Here's how the part is built. I have some questions about the finished solid (model axes, mm). Face numbers are marked on the shaded views. A direction names the side the tool comes from. Round coordinates to 2 decimals unless told otherwise and drop trailing zeros. Write each loop counter-clockwise with the first axis right and the second up, starting at its lowest first coordinate (ties: lowest second). Pieces come first, ordered by that corner, then holes. Notation, with made-up numbers: (-29, -24.75) - (1, -24.75) arc R27 cw to (1, 2.25) - close; hole circle Ø3 at (9.25, 58). An arc over 180 degrees is marked (long way). Return JSON: item names as keys, results as strings. Group by question number.
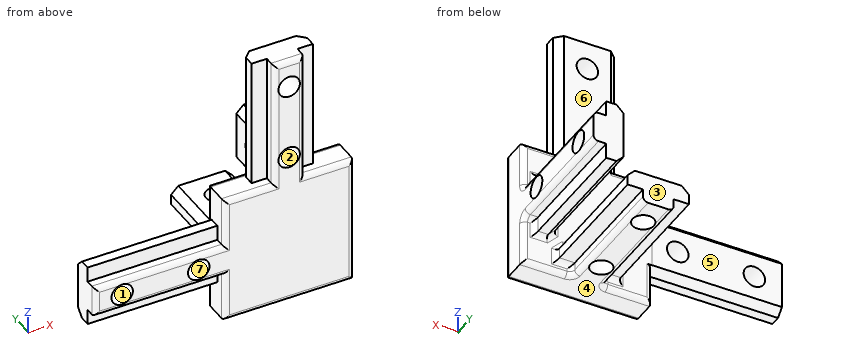
```python
from build123d import *

# Parameters (mm, degrees)
SKETCH1_W             = 25.4
SKETCH1_H             = 25.4
BOSS_EXTRUDE1_DEPTH   = 5.91
BOSS_EXTRUDE2_DEPTH   = 25.4
BOSS_EXTRUDE3_DEPTH   = 25.4
BOSS_EXTRUDE4_DEPTH   = 25.4
FILLET2_R             = 1
M5X0_8_TAPPED_HOLE2_D = 4.2
M5X0_8_TAPPED_HOLE3_D = 4.2
M5X0_8_TAPPED_HOLE4_D = 4.2


with BuildPart() as part:
    # Sketch1 → Boss-Extrude1 (new body)
    with BuildSketch(Plane(origin=(0, 0, 0), x_dir=(1, 0, 0), z_dir=(0, 1, 0))):
        Rectangle(SKETCH1_W, SKETCH1_H)
    extrude(amount=BOSS_EXTRUDE1_DEPTH)

    # Sketch2 → Boss-Extrude2 (add)
    with BuildSketch(Plane.XY.offset(12.7)):
        Polygon((-3, 0), (3, 0), (3, 2.5), (6, 2.5), (6, 4.5), (4.585786438, 5.914213562), (-4.585786438, 5.914213562), (-6, 4.5), (-6, 2.5), (-3, 2.5), align=None)
    extrude(amount=BOSS_EXTRUDE2_DEPTH)

    # Sketch3 → Boss-Extrude3 (add)
    with BuildSketch(Plane.ZY.offset(12.7)):
        Polygon((-3, 0), (3, 0), (3, 2.5), (6, 2.5), (6, 4.5), (4.585786438, 5.914213562), (-4.585786438, 5.914213562), (-6, 4.5), (-6, 2.5), (-3, 2.5), align=None)
    extrude(amount=BOSS_EXTRUDE3_DEPTH)

    # Sketch5 → Boss-Extrude4 (add)
    with BuildSketch(Plane(origin=(0, 5.91, 0), x_dir=(1, 0, 0), z_dir=(0, 1, 0))):
        Polygon((3, 12.7), (-3, 12.7), (-3, 10.2), (-6, 10.2), (-6, 8.2), (-4.585786438, 6.785786438), (4.585786438, 6.785786438), (6, 8.2), (6, 10.2), (3, 10.2), align=None)
        Polygon((12.7, -3), (12.7, 3), (10.2, 3), (10.2, 6), (8.2, 6), (6.785786438, 4.585786438), (6.785786438, -4.585786438), (8.2, -6), (10.2, -6), (10.2, -3), align=None)
    extrude(amount=BOSS_EXTRUDE4_DEPTH)

    # Fillet2
    fillet2_edges = [part.edges().sort_by_distance(p)[0] for p in [
        (7.492893219, 5.91, -5.292893219),
        (6.785786438, 5.91, 0),
        (7.492893219, 5.91, 5.292893219),
        (9.2, 5.91, 6),
        (10.2, 5.91, 4.5),
        (11.45, 5.91, 3),
        (12.7, 18.61, 3),
        (-12.7, 5.91, -8.645),
        (7.85, 0, 12.7),
        (8.645, 5.91, 12.7),
        (-8.645, 5.91, 12.7),
        (3, 0, 25.4),
        (-3, 0, 25.4),
        (0, 0, 38.1),
        (-12.7, 0, 7.85),
        (-12.7, 5.91, 8.645),
        (-25.4, 0, 3),
        (12.7, 5.91, 7.85),
        (-7.85, 0, 12.7),
        (-12.7, 0, -7.85),
        (-25.4, 0, -3),
        (-38.1, 0, 0),
        (0, 0, -12.7),
        (12.7, 0, 0),
        (12.7, 5.91, -7.85),
        (-7.85, 5.91, -12.7),
        (-3, 5.91, -11.45),
        (-3, 18.61, -12.7),
        (-4.5, 5.91, -10.2),
        (-6, 5.91, -9.2),
        (-5.292893219, 5.91, -7.492893219),
        (0, 5.91, -6.785786438),
        (5.292893219, 5.91, -7.492893219),
        (6, 5.91, -9.2),
        (4.5, 5.91, -10.2),
        (3, 5.91, -11.45),
        (3, 18.61, -12.7),
        (7.85, 5.91, -12.7),
        (11.45, 5.91, -3),
        (12.7, 18.61, -3),
        (10.2, 5.91, -4.5),
        (9.2, 5.91, -6),
    ]]
    fillet(fillet2_edges, radius=FILLET2_R)

    # M5x0.8 Tapped Hole2 (through all)
    with Locations(Plane(origin=(0, 0, 0), x_dir=(-1, 0, 0), z_dir=(0, -1, 0))):
        with Locations((0, -17.7), (0, -32.7), (17.7, 0), (32.7, 0)):
            Hole(M5X0_8_TAPPED_HOLE2_D / 2)

    # M5x0.8 Tapped Hole3 (through all)
    with Locations(Plane(origin=(12.7, 0, 0), x_dir=(0, 0, -1), z_dir=(1, 0, 0))):
        with Locations((0, 10.91), (0, 25.91)):
            Hole(M5X0_8_TAPPED_HOLE3_D / 2)

    # M5x0.8 Tapped Hole4 (through all)
    with Locations(Plane(origin=(0, 0, -12.7), x_dir=(-1, 0, 0), z_dir=(0, 0, -1))):
        with Locations((0, 25.91), (0, 10.91)):
            Hole(M5X0_8_TAPPED_HOLE4_D / 2)


solid = part.part
```
1) Imagine slicing it at A-A (y = 14.5). Please give me the cut outline in (x, z).
2) For the marked faces 5, 6 and 7, which set-ups out of +Z, -Z, +X, -X, +Y, -Y let a thin tool reach every point of the face, with its end or its side?
3) Imagine slicing it at B-B (x = 0). Give the number of separate pieces and of enclosed holes in the cut face, plus the area to 3 significant figures.
4) Will these pins go through, and if not, where does the flat tip stop? pin 1 Ø3 at (x, z) = (-18, -5) entering from -Y; pin 2 Ø2 at (x, z) = (-3.5, -6) entering from +Y; pin 3 Ø2 at (x, y) = (-8.5, 2.5) entering from +Z; pin 4 Ø1 at (y, z) = (4, 19.5) entering from -X.
5) Imagine slicing it at D-D (z = 17.7). Please give me the cut outline in (x, y).
6) If we mould it in two halves opening along Z, with no side actions, what happens to the marked faces 1, 2, 3 and 4? For each: released by +Z, released by -Z, zero draft, split by the parting line, or undercut.
7) I need wall thicknesses on line 1 along Z through (x, y) = (0, 4.5); line 2 along Z through (x, y) = (-32.7, 1.45); line 3 along Y through (x, z) = (-1, -2). Which ranges of each line are inside material? Lowest first, please.
Results found:
{
 "1": {"outline": "(-6, -10.2) - (-3, -10.2) - (-3, -11.7) arc R1 ccw to (-2, -12.7) - (2, -12.7) arc R1 ccw to (3, -11.7) - (3, -10.2) - (6, -10.2) - (6, -8.2) - (4.59, -6.79) - (-4.59, -6.79) - (-6, -8.2) - close; (6.79, -4.59) - (8.2, -6) - (10.2, -6) - (10.2, -3) - (11.7, -3) arc R1 ccw to (12.7, -2) - (12.7, 2) arc R1 ccw to (11.7, 3) - (10.2, 3) - (10.2, 6) - (8.2, 6) - (6.79, 4.59) - close"},
 "2": {"face 5": "+Z, -Z, -X, +Y", "face 6": "+Z, +X, -X, +Y", "face 7": "+Y, -Y"},
 "3": {"separate pieces": "5", "enclosed holes": "0", "area": "351 mm²"},
 "4": {"pin 1": "stops at y = 2.5", "pin 2": "stops at y = 31.31", "pin 3": "stops at z = 12.7", "pin 4": "stops at x = -6"},
 "5": {"outline": "(-6, 2.5) - (-3, 2.5) - (-3, 1) arc R1 ccw to (-2.1, 0.01) - (-2.1, 5.91) - (-4.59, 5.91) - (-6, 4.5) - close; (2.1, 0.01) arc R1 ccw to (3, 1) - (3, 2.5) - (6, 2.5) - (6, 4.5) - (4.59, 5.91) - (2.1, 5.91) - close"},
 "6": {"face 1": "undercut", "face 2": "undercut", "face 3": "zero draft", "face 4": "released by -Z"},
 "7": {"line 1": "z = -12.7 to 15.6, 19.8 to 30.6, 34.8 to 38.1", "line 2": "z = -3 to -2.1, 2.1 to 3", "line 3": "y = 0 to 5.91"}
}
